Verification items for the finished model (mm, model axes). Face numbers are marked on the shaded views. Round coordinates to 2 decimals unless told otherwise and drop trailing zeros. Order: outer loops, then holes, each group sorted by start corner. A loop starts at its lowest first (then second) coordinate and runs counter-clockwise, first axis right, second up. Notation, with made-up numbers: (58, 75.5) -> (65, 75.5) arc R20 ccw to (65, 104.5) -> close; hole circle Ø8 at (-5.5, 39.25). An arc over 180 degrees is marked (long way). Put each result on its own line as item: value.
```python
from build123d import *

# Parameters (mm, degrees)
SKETCH1_W           = 27
SKETCH1_H           = 8
SKETCH1_R           = 1.6
BOSS_EXTRUDE1_DEPTH = 1.7
FILLET1_R           = 0.5
FILLET2_R           = 0.5


with BuildPart() as part:
    # Sketch1 → Boss-Extrude1 (new body)
    with BuildSketch(Plane(origin=(0, 0, 0), x_dir=(1, 0, 0), z_dir=(0, 1, 0))):
        Rectangle(SKETCH1_W, SKETCH1_H)
        with Locations((-10.75, 0)):
            Circle(SKETCH1_R, mode=Mode.SUBTRACT)
        with Locations((10.75, 0)):
            Circle(SKETCH1_R, mode=Mode.SUBTRACT)
    extrude(amount=BOSS_EXTRUDE1_DEPTH)

    # Fillet1
    fillet1_edges = [part.edges().sort_by_distance(p)[0] for p in [
        (0, 0, -4),
        (13.5, 0, 0),
        (0, 0, 4),
        (-13.5, 0, 0),
    ]]
    fillet(fillet1_edges, radius=FILLET1_R)

    # Fillet2
    fillet2_edges = [part.edges().sort_by_distance(p)[0] for p in [
        (13.5, 1.7, 0),
        (0, 1.7, -4),
        (-13.5, 1.7, 0),
        (0, 1.7, 4),
    ]]
    fillet(fillet2_edges, radius=FILLET2_R)


solid = part.part
```
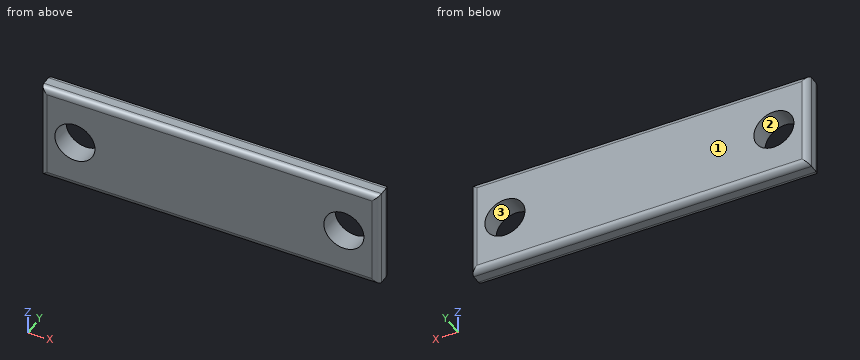
Item 1: Sectioned sample at B-B, the plane z = 0. Record the boundary of the cut face in (x, y), then the cut area to 3 significant figures.
Geometry check:
outline: (-13.5, 0.5) arc R0.5 ccw to (-13, 0) -> (-12.35, 0) -> (-12.35, 1.7) -> (-13, 1.7) arc R0.5 ccw to (-13.5, 1.2) -> close; (-9.15, 0) -> (9.15, 0) -> (9.15, 1.7) -> (-9.15, 1.7) -> close; (12.35, 0) -> (13, 0) arc R0.5 ccw to (13.5, 0.5) -> (13.5, 1.2) arc R0.5 ccw to (13, 1.7) -> (12.35, 1.7) -> close
area: 34.8 mm2
Item 2: Sectioned sample at C-C, the plane y = 0.9. Record the boundary of the cut face in (x, z), then the cut area to 3 significant figures.
Geometry check:
outline: (-13.5, -4) -> (13.5, -4) -> (13.5, 4) -> (-13.5, 4) -> close; hole circle Ø3.2 at (-10.75, 0); hole circle Ø3.2 at (10.75, 0)
area: 200 mm2
Item 3: Sectioned sample at A-A, the plane x = 10.75. Record the boundary of the cut face in (y, z), then the cut area to 3 significant figures.
Geometry check:
outline: (0, -3.5) arc R0.5 ccw to (0.5, -4) -> (1.2, -4) arc R0.5 ccw to (1.7, -3.5) -> (1.7, -1.6) -> (0, -1.6) -> close; (0, 1.6) -> (1.7, 1.6) -> (1.7, 3.5) arc R0.5 ccw to (1.2, 4) -> (0.5, 4) arc R0.5 ccw to (0, 3.5) -> close
area: 7.95 mm2
Item 4: Sectioned sample at D-D, the plane x = 4.5. Record the boundary of the cut face in (y, z), then the cut area to 3 significant figures.
Geometry check:
outline: (0, -3.5) arc R0.5 ccw to (0.5, -4) -> (1.2, -4) arc R0.5 ccw to (1.7, -3.5) -> (1.7, 3.5) arc R0.5 ccw to (1.2, 4) -> (0.5, 4) arc R0.5 ccw to (0, 3.5) -> close
area: 13.4 mm2
Item 5: Material ranges on line 1 along X through (y, z) = (1.25, 0); line 2 along Z through (x, y) = (10.75, 1.05); line 3 along X through (y, z) = (1.55, 1), recorded low to high.
Geometry check:
line 1: -13.5 to -12.35, -9.15 to 9.15, 12.35 to 13.5
line 2: -4 to -1.6, 1.6 to 4
line 3: -13.36 to -12, -9.5 to 9.5, 12 to 13.36
Item 6: Release check for a two-part mould opening along Z. For the marked faces 1, 2 and 3 record: pulls with the +Z half, pulls with the -Z half, needs draft (parallel to the pull), parting line crosses it, or undercut.
Geometry check:
face 1: needs draft
face 2: undercut
face 3: undercut
